The listing builds one solid part. Answer for the finished solid, in the listing's coordinates (mm). A direction names the side the tool comes from. Coordinates: 2 decimals unless noted, no trailing zeros. Write each loop counter-clockwise with the first axis right and the second up, starting at its lowest first coordinate (ties: lowest second). Pieces come first, ordered by that corner, then holes. Notation, with made-up numbers: M 62,82 L 83,82 A33 cw 83,118 Z; hole C -15.5,41.25 d2. An arc over 180 degrees is marked long. Answer as CSV lines item,"result".
Autodesk Inventor part; units mm, degrees
ref_plane "YZ Plane" through (0, 0, 0) normal (1, 0, 0) x (0, 1, 0)
ref_plane "XZ Plane" through (0, 0, 0) normal (0, 1, 0) x (-1, 0, 0)
ref_plane "XY Plane" through (0, 0, 0) normal (0, 0, 1) x (1, 0, 0)
sketch "Szkic1" plane through (0, 0, 0) normal (0, 1, 0) x (-1, 0, 0)
  circle A0 centre (0, 0) radius 5
  line L0 (-6, 6.5) -> (6, 6.5)
  line L1 (6, 6.5) -> (6, -6.5)
  line L2 (6, -6.5) -> (-6, -6.5)
  line L3 (-6, -6.5) -> (-6, 6.5)
  line L4 (-6, 6.5) -> (6, -6.5) construction
  line L5 (6, 6.5) -> (-6, -6.5) construction
  line L6 (6, 6.5) -> (18, 6.5)
  line L7 (18, 6.5) -> (18, 3.5)
  line L8 (18, 3.5) -> (6, 3.5)
  line L9 (6, 3.5) -> (6, 6.5)
  line L10 (6, -6.5) -> (18, -6.5)
  line L11 (18, -6.5) -> (18, -3.5)
  line L12 (18, -3.5) -> (6, -3.5)
  line L13 (6, -3.5) -> (6, -6.5)
  dimension "d0" = 10
  dimension "d1" = 12
  dimension "d2" = 13
  dimension "d8" = 12
  dimension "d9" = 3
  dimension "d10" = 3
extrude "Wyciągnięcie proste1" add sketch "Szkic1" along normal blind 10
thread "Gwint1"
sketch "Szkic2" plane through (-18, 0, 6.5) normal (0, 0, 1) x (1, 0, 0)
  line L0 (0, 0) -> (0, 10)
  line L1 (12, 0) -> (12, 10)
  circle A0 centre (5, 5) radius 4.1
  line L2 (0, 0) -> (24, 0)
  point P0 (18, 0)
  dimension "d11" = 8.2
  dimension "d16" = 7
  dimension "d17" = 5
extrude "Wyciągnięcie proste2" cut sketch "Szkic2" against normal blind 16.75
fillet "Zaokrąglenie2" radius 3 4 edges at (-18, 10, -5) (-18, 0, -5) (-18, 0, 5) (-18, 10, 5)
properties part number "konik"
Q1. Find section D-D (z = 0). Give the vertices of the cut face in (x, y).
Output:
outline,"M -6,0 L -5,0 L -5,10 L -6,10 Z; M 5,0 L 6,0 L 6,10 L 5,10 Z"
Q2. Find section A-A (y = 5). Give the vertices of the cut face in (x, z).
Output:
outline,"M -18,-6.5 L -17.1,-6.5 L -17.1,-3.5 L -18,-3.5 Z; M -18,3.5 L -17.1,3.5 L -17.1,6.5 L -18,6.5 Z; M -8.9,-6.5 L 6,-6.5 L 6,6.5 L -8.9,6.5 L -8.9,3.5 L -6,3.5 L -6,-3.5 L -8.9,-3.5 Z; hole C 0,0 d10"
Q3. Flat-ended cylindrical pins translate along their axes: pin 1 Ø2 at (y, z) = (4.5, -0.5) entering from -X; pin 2 Ø3 at (x, y) = (-11, 4) entering from +Z. Find the tip coordinate at first contact, or state that the pin passes through.
Output:
pin 1,"x = -6"
pin 2,"through"
Q4. Find section C-C (x = 0). Give the vertices of the cut face in (y, z), and give its area (3 significant figures).
Output:
outline,"M 0,-6.5 L 10,-6.5 L 10,-5 L 0,-5 Z; M 0,5 L 10,5 L 10,6.5 L 0,6.5 Z"
area,"30.0 mm2"
Q5. Straight lines are drawn through the part: line 1 (Z direction, x = -9.5, y = 2); line 2 (Y direction, x = -13, z = -4.55); line 3 (Z direction, x = 0, y = 2). For each, find the intervals that lie inside material, in ascending order.
Output:
line 1,"-6.5 to -3.5, 3.5 to 6.5"
line 2,"0 to 0.9, 9.1 to 10"
line 3,"-6.5 to -5, 5 to 6.5"
Q6. Find section B-B (z = -4). Give the vertices of the cut face in (x, y), and give its area (3 significant figures).
Output:
outline,"M -18,3 A3 ccw -15,0 L -3,0 L -3,10 L -15,10 A3 ccw -18,7 Z; M 3,0 L 6,0 L 6,10 L 3,10 Z; hole C -13,5 d8.2"
area,"123 mm2"
Q7. For faces 1 (the flat face through (-9, 7, -3.5)), 2 (the flat face through (6, 5, 0)), determine the directions among +Z, -Z, +X, -X, +Y, -Y from which every point of the face is accessible in a straight line to the end or side of a thin tool.
Output:
face 1,"-X, +Y, -Y"
face 2,"+Z, -Z, +X, +Y, -Y"
Q8. The mould has two halves that part along Z. Classify faces 3 (the flat face through (-3, 5, 6.5)), 4 (the flat face through (-9, 7, 3.5)), 5 (the flat face through (-18, 5, -5)): pulls with the +Z half, pulls with the -Z half, needs draft (parallel to the pull), parting line crosses it, or undercut.
Output:
face 3,"pulls with the +Z half"
face 4,"undercut"
face 5,"needs draft"
